Solid Edge part; units mm, degrees
sketch "Sketch1" plane through (0, 0, 0) normal (0, 0, 1) x (1, 0, 0)
  line L0 (-7.4, -3.75) -> (7.4, -3.75)
  arc A0 (7.4, -3.75) -> (11.15, 0) centre (7.4, 0) ccw
  arc A1 (11.15, 0) -> (7.4, 3.75) centre (7.4, 0) ccw
  line L1 (7.4, 3.75) -> (-7.4, 3.75)
  arc A2 (-7.4, 3.75) -> (-11.15, 0) centre (-7.4, 0) ccw
  arc A3 (-7.4, -3.75) -> (-11.15, 0) centre (-7.4, 0) cw
  dimension "D1" = 7.4
extrude "Protrusion1" add sketch "Sketch1" along normal mid plane 4.7
sketch "Sketch2" plane through (0, 0, 2.35) normal (0, 0, 1) x (1, 0, 0)
  line L0 (-7.4, -2.75) -> (7.4, -2.75)
  arc A0 (7.4, -2.75) -> (10.15, 0) centre (7.4, 0) ccw
  arc A1 (10.15, 0) -> (7.4, 2.75) centre (7.4, 0) ccw
  line L1 (7.4, 2.75) -> (-7.4, 2.75)
  arc A2 (-7.4, 2.75) -> (-10.15, 0) centre (-7.4, 0) ccw
  arc A3 (-7.4, -2.75) -> (-10.15, 0) centre (-7.4, 0) cw
  dimension "D1" = 7.4
extrude "Extrusionsausschnitt_1" cut sketch "Sketch2" against normal blind 1.2 flip side to cut
sketch "Sketch3" plane through (0, 0, -2.35) normal (0, 0, -1) x (1, 0, 0)
  line L0 (-7.4, -2.75) -> (7.4, -2.75)
  arc A0 (7.4, -2.75) -> (10.15, 0) centre (7.4, 0) ccw
  arc A1 (10.15, 0) -> (7.4, 2.75) centre (7.4, 0) ccw
  line L1 (7.4, 2.75) -> (-7.4, 2.75)
  arc A2 (-7.4, 2.75) -> (-10.15, 0) centre (-7.4, 0) ccw
  arc A3 (-7.4, -2.75) -> (-10.15, 0) centre (-7.4, 0) cw
  dimension "D1" = 7.4
extrude "Extrusionsausschnitt_2" cut sketch "Sketch3" against normal blind 2.5 flip side to cut
sketch "Sketch4" plane through (0, 0, 2.35) normal (0, 0, 1) x (1, 0, 0)
  line L0 (-2.56, -1.76) -> (4.32, -1.76)
  line L1 (4.32, -1.76) -> (4.32, 1.76)
  line L2 (4.32, 1.76) -> (-2.56, 1.76)
  arc A0 (-2.56, 1.76) -> (-4.32, 0) centre (-2.56, 0) ccw
  arc A1 (-2.56, -1.76) -> (-4.32, 0) centre (-2.56, 0) cw
  dimension "D1" = 4.32
  dimension "D2" = 4.32
extrude "Extrusionsausschnitt_3" cut sketch "Sketch4" against normal blind 1.2
fillet "Verrundung_1" radius 0.1 11 edges at (0, 3.75, 1.15) (-11.15, 0, 1.15) (0, -3.75, 1.15) (0, 2.75, 2.35) (-10.15, 0, 2.35) (0, -2.75, 2.35) (10.15, 0, 2.35) (-4.32, 0, 2.35) (0.88, -1.76, 2.35) (0.88, 1.76, 2.35) (4.32, 0, 2.35)
sketch "Sketch5" plane through (0, 0, 1.15) normal (0, 0, 1) x (1, 0, 0)
  circle A0 centre (-2.56, 0) radius 0.5
  circle A1 centre (-0.06, 0) radius 0.5
  circle A2 centre (2.44, 0) radius 0.5
extrude "Extrusionsausprägung_2" add sketch "Sketch5" along normal blind 1 and the other way blind 5
CAD build for the part. Positions are in the model's coordinates, mm. A direction names the side the tool comes from. Round coordinates to 2 decimals unless told otherwise and drop trailing zeros. Write each loop counter-clockwise with the first axis right and the second up, starting at its lowest first coordinate (ties: lowest second). Pieces come first, ordered by that corner, then holes.
Item 1: Mould opens along Y. For faces 4 (the flat face through (-0.1, -2.3, 2.35)), 5 (the flat face through (0, 0, 2.15)), 6 (the flat face through (0, 2.75, 2)) say: released by +Y, released by -Y, zero draft, split by the parting line, or undercut.
Filled in:
face 4: zero draft
face 5: undercut
face 6: released by +Y
Item 2: Drop flat-ended pins along their axis: pin 1 Ø0.8 at (x, z) = (-1, -1.5) entering from +Y; pin 2 Ø0.8 at (x, y) = (-2.5, 0) entering from +Z; pin 3 Ø1.6 at (x, y) = (3.5, 0.5) entering from -Z; pin 4 Ø3 at (x, y) = (3, -2.5) entering from -Z. Give the stop position or say it passes through.
Filled in:
pin 1: stops at y = 2.75
pin 2: stops at z = 2.15
pin 3: stops at z = -3.85
pin 4: stops at z = -2.35
Item 3: Drill centre lines: L1, parallel to Z at x = 0.25, y = -1.5; L2, parallel to Y at x = 5.75, z = 0; L3, parallel to Z at x = 4, y = 3.25. Where is each one in solid material? Low to high.
Filled in:
L1: z = -2.35 to 1.15
L2: y = -2.75 to 2.75
L3: z = 0.15 to 1.15
Item 4: Tool access for faces 1 (the cylindrical face through (10.15, -0.06, 1.71)), 2 (the cylindrical face through (-2.1, -0.2, -3.1)), 3 (the cylindrical face through (-4.32, 0.04, 1.71)): list every direction of +Z, -Z, +X, -X, +Y, -Y with a clear straight run to the whole face (end or side of a thin tool).
Filled in:
face 1: +Z, +X
face 2: -Z
face 3: +Z
Item 5: Band-saw the part on B-B on x = 6. Write the cut outline in (y, z).
Filled in:
outline: (-3.75, 0.15) - (-2.75, 0.15) - (-2.75, -2.35) - (2.75, -2.35) - (2.75, 0.15) - (3.75, 0.15) - (3.75, 1.05) arc R0.1 ccw to (3.65, 1.15) - (2.75, 1.15) - (2.75, 2.25) arc R0.1 ccw to (2.65, 2.35) - (-2.65, 2.35) arc R0.1 ccw to (-2.75, 2.25) - (-2.75, 1.15) - (-3.65, 1.15) arc R0.1 ccw to (-3.75, 1.05) - close
